Geometry: final body of the model. Coordinates: model frame, mm. A direction names the side the tool comes from. Give positions to 0.01 mm unless a question says otherwise; leave off trailing zeros. Write each loop counter-clockwise with the first axis right and the second up, starting at its lowest first coordinate (ties: lowest second). Pieces come first, ordered by that corner, then holes. Notation, with made-up numbers: (72.5, 14) - (108.5, 14) arc R15 ccw to (108.5, 40) - close; hole circle Ø6 at (17, 42.25). An arc over 180 degrees is marked (long way). One line per question, with ' | ' between items. Start each with the question number.
Autodesk Inventor part; units mm, degrees
ref_plane "YZ Plane" through (0, 0, 0) normal (1, 0, 0) x (0, 1, 0)
ref_plane "XZ Plane" through (0, 0, 0) normal (0, 1, 0) x (-1, 0, 0)
ref_plane "XY Plane" through (0, 0, 0) normal (0, 0, 1) x (1, 0, 0)
sketch "Эскиз1" plane through (0, 0, 0) normal (0, 0, 1) x (1, 0, 0)
  line L0 (-11.5, -21.5) -> (11.7, -21.5)
  line L1 (11.7, -21.5) -> (11.7, 19.5)
  line L2 (11.7, 19.5) -> (-11.5, 19.5)
  line L3 (-11.5, 19.5) -> (-11.5, -21.5)
  circle A0 centre (-9, -10.5) radius 1.5
  point P0 (0, 0)
  dimension "d0" = 23.2
  dimension "d1" = 41
  dimension "d4" = 11
  dimension "d5" = 2.5
extrude "Выдавливание1" add sketch "Эскиз1" along normal blind 1.7 contours L3 L2 L1 L0 | A0
sketch "Эскиз2" plane through (0, 0, 1.7) normal (0, 0, 1) x (1, 0, 0)
  circle A0 centre (-9, -9.9846) radius 1.5
  circle A1 centre (9, -9.9846) radius 1.5
  circle A2 centre (-9, 11.0154) radius 1.5
  circle A3 centre (9, 11.0154) radius 1.5
  point P0 (0, 0)
extrude "Выдавливание2" cut sketch "Эскиз2" against normal blind 1.7
sketch "Эскиз3" plane through (0, 0, 1.7) normal (0, 0, 1) x (1, 0, 0)
  line L0 (-9, -21.5) -> (9, -21.5)
  line L1 (9, -21.5) -> (9, -13.3)
  line L2 (9, -13.3) -> (-9, -13.3)
  line L3 (-9, -13.3) -> (-9, -21.5)
  line L4 (-11.5, -21.5) -> (11.7, -21.5)
  point P0 (0, 0)
  point P1 (0, -21.5)
  point P2 (0.1, -21.5)
  dimension "d8" = 18
  dimension "d9" = 8.2
extrude "Выдавливание3" add sketch "Эскиз3" along normal blind 5.6
sketch "Эскиз4" plane through (-11.5, -21.5, 0) normal (0, -1, 0) x (1, 0, 0)
  circle A0 centre (6, 3.65) radius 0.6
  line L0 (2.5, 7.3) -> (20.5, 7.3)
  line L1 (6, 7.3) -> (6, 0) construction
  line L2 (0, 0) -> (0, 1.7)
  circle A1 centre (7.8, 3.65) radius 0.6
  circle A2 centre (9.6, 3.65) radius 0.6
  circle A3 centre (11.4, 3.65) radius 0.6
  circle A4 centre (13.2, 3.65) radius 0.6
  circle A5 centre (15, 3.65) radius 0.6
  circle A6 centre (16.8, 3.65) radius 0.6
  point P0 (11.5, 0)
  dimension "d12" = 1.2
  dimension "d13" = 6
  dimension "d16" = 1.8
extrude "Выдавливание4" add sketch "Эскиз4" along normal blind 12.6
sketch "Эскиз5" plane through (0, 0, 1.7) normal (0, 0, 1) x (1, 0, 0)
  line L0 (-7.65, 12.3) -> (7.85, 12.3)
  line L1 (7.85, 12.3) -> (7.85, 19.5)
  line L2 (7.85, 19.5) -> (-7.65, 19.5)
  line L3 (-7.65, 19.5) -> (-7.65, 12.3)
  line L4 (11.7, 19.5) -> (-11.5, 19.5)
  point P0 (0, 0)
  point P1 (0.1, 19.5)
  point P2 (0.1, 19.5)
  dimension "d23" = 15.5
  dimension "d24" = 7.2
extrude "Выдавливание5" add sketch "Эскиз5" along normal blind 2.1
sketch "Эскиз6" plane through (-11.5, 19.5, 0) normal (0, 1, 0) x (1, 0, 0)
  line L0 (17.75, -3.5) -> (5.25, -3.5)
  line L1 (5.25, -3.5) -> (5.25, -3.4)
  line L2 (5.25, -3.4) -> (17.75, -3.4)
  line L3 (17.75, -3.4) -> (17.75, -3.5)
  line L4 (20.5, -7.3) -> (2.5, -7.3)
  line L5 (19.35, -3.8) -> (3.85, -3.8)
  point P0 (11.5, 0)
  point P1 (11.5, -3.4)
  point P2 (11.5, -7.3)
  dimension "d27" = 12.5
  dimension "d28" = 0.1
  dimension "d29" = 0.3
sketch "Эскиз7" plane through (0, 0, 0) normal (1, 0, 0) x (0, 1, 0)
  line L0 (19.5, 3.4) -> (19.5, 3.5)
  line L1 (20.262, -17.8921) -> (54.1609, -17.8921) construction
  arc A0 (19.5, 3.5) -> (40.8268, 24.8268) centre (19.5, 24.8268) ccw
  line L2 (19.5, 1.7) -> (19.5, 3.8)
  line L3 (31.9208, 24.8268) -> (55.6437, 24.8268) construction
  point P0 (0, 0)
  dimension "d40" = 33.5
sweep "Сдвиг1" add profiles "Эскиз6" path "Эскиз7" path curves A0
ref_plane "РабПлоскость2" through (0, 40.768, -17.8921) normal (0, 1, 0) x (-1, 0, 0)
sketch "Эскиз9" plane through (0, 40.768, -17.8921) normal (0, 1, 0) x (-1, 0, 0)
  line L0 (21, 70.2189) -> (-21, 70.2189)
  line L1 (-21, 70.2189) -> (-21, 42.7189)
  line L2 (-21, 42.7189) -> (21, 42.7189)
  line L3 (21, 42.7189) -> (21, 70.2189)
  line L4 (-6.25, 42.7189) -> (6.25, 42.7189)
  point P0 (0, 17.8921)
  point P1 (0, 42.7189)
  dimension "d41" = 42
  dimension "d42" = 27.5
extrude "Выдавливание6" add sketch "Эскиз9" along normal blind 0.15
properties part number "ЛЦМК000002.00.00.00.00.13 OLED"
1) First-contact query: pin 1 Ø1 at (x, y) = (7, -21.5) entering from +Z; pin 2 Ø1.9 at (y, z) = (4, 0.5) entering from -X; pin 3 Ø6 at (y, z) = (-19, 4.5) entering from +X. Flat tips, straight axial feed; report the tip coordinate or a pass-through.
2) Line query: L1, parallel to Y at x = 9, z = 1.3; L2, parallel to Z at x = -9, y = 18; L3, parallel to Z at x = 7, y = -18. Output: solid intervals per line, ascending.
3) Section B-B, the plane z = 41.5. Output: boundary loops of the cut face in (x, y), plus the area to 3 significant figures.
4) Pull-direction query (Y, two-part tool) for faces 1 (the cylindrical face through (7.81, -10.9, 0.86)), 2 (the flat face through (-9, -17, 4)), 3 (the flat face through (0, -1, 1.7)), 4 (the flat face through (-0.1, -21.5, 2.8)); classes: +Y half, -Y half, draft (parallel to the pull), parting line (faces both ways), or undercut.
5) Section A-A, the plane y = 7.5. Output: boundary loops of the cut face in (x, z), plus the area to 3 significant figures.
6) Reachability of faces 5 (the flat face through (-7.65, 16, 3)), 6 (the flat face through (9, -17, 4)), 7 (the flat face through (0, 16, 3.8)) from +Z, -Z, +X, -X, +Y, -Y: full face, straight path, thin tool, end or side. Return the list, or none.
Answer key:
1) pin 1: z = 7.3 | pin 2: x = -11.5 | pin 3: x = 11.7
2) L1: -21.5 to -11.48, -8.48 to 9.52, 12.52 to 19.5 | L2: 0 to 1.7 | L3: 0 to 7.3
3) outline: (-21, 40.77) - (21, 40.77) - (21, 40.92) - (-21, 40.92) - close | area: 6.30 mm^2
4) face 1: undercut | face 2: draft | face 3: undercut | face 4: -Y half
5) outline: (-11.5, 0) - (11.7, 0) - (11.7, 1.7) - (-11.5, 1.7) - close | area: 39.4 mm^2
6) face 5: +Z, -X, +Y | face 6: +Z, +X, +Y, -Y | face 7: +Z, +X, -X
